```python
from build123d import *

# Parameters (mm, degrees)
F1_DEPTH       = 75
F2_T           = -0.01
F5_DEPTH       = 10
F6_DEPTH       = 10
F7_DEPTH       = 10
F8_DEPTH       = 10
F9_DEPTH       = 10
F10_DEPTH      = 10
F11_DEPTH      = 10
F12_DEPTH      = 10
F13_DEPTH      = 5
F4_E8_BOTTOM_W = 32
F4_E8_BOTTOM_H = 28
F14_DEPTH      = 0.01
F15_DEPTH      = 68


with BuildPart() as f1:
    # F0 (on Top) → F1 (new body)
    with BuildSketch(Plane.XY):
        Polygon((0, -147), (0, 0), (-70, 0), (-70, -45), (-135, -45), (-135, -96), (-120, -96), (-120, -147), align=None)
    extrude(amount=F1_DEPTH)

    # F2
    f2_openings = [f1.faces().sort_by_distance(p)[0] for p in [
        (-58.321727, -80.461003, 75),
    ]]
    offset(amount=F2_T, openings=f2_openings, kind=Kind.INTERSECTION)

    # F5 (add): a face of the model
    f5_faces = [f1.faces().sort_by_distance(p)[0] for p in [
        (0, -73.5, 37.5),
    ]]
    extrude(f5_faces, amount=F5_DEPTH)

    # F6 (add): a face of the model
    f6_faces = [f1.faces().sort_by_distance(p)[0] for p in [
        (-30, 0, 37.5),
    ]]
    extrude(f6_faces, amount=F6_DEPTH)

    # F7 (add): a face of the model
    f7_faces = [f1.faces().sort_by_distance(p)[0] for p in [
        (-70, -17.5, 37.5),
    ]]
    extrude(f7_faces, amount=F7_DEPTH)

    # F8 (add): a face of the model
    f8_faces = [f1.faces().sort_by_distance(p)[0] for p in [
        (-107.5, -45, 37.5),
    ]]
    extrude(f8_faces, amount=F8_DEPTH)

    # F9 (add): a face of the model
    f9_faces = [f1.faces().sort_by_distance(p)[0] for p in [
        (-135, -65.5, 37.5),
    ]]
    extrude(f9_faces, amount=F9_DEPTH)

    # F10 (add): a face of the model
    f10_faces = [f1.faces().sort_by_distance(p)[0] for p in [
        (-132.5, -96, 37.5),
    ]]
    extrude(f10_faces, amount=F10_DEPTH)

    # F11 (add): a face of the model
    f11_faces = [f1.faces().sort_by_distance(p)[0] for p in [
        (-120, -126.5, 37.5),
    ]]
    extrude(f11_faces, amount=F11_DEPTH)

    # F12 (add): a face of the model
    f12_faces = [f1.faces().sort_by_distance(p)[0] for p in [
        (-60, -147, 37.5),
    ]]
    extrude(f12_faces, amount=F12_DEPTH)

    # F13 (add): a face of the model
    f13_faces = [f1.faces().sort_by_distance(p)[0] for p in [
        (-59.1569047083, -79.5398738455, 0),
    ]]
    extrude(f13_faces, amount=F13_DEPTH)

    # F4_E8_bottom (on explicit) → F14 (join, through all)
    with BuildSketch(Plane(origin=(-134, -45, 0), x_dir=(1, 0, 0), z_dir=(0, 0, -1))):
        with Locations((16, 14)):
            Rectangle(F4_E8_BOTTOM_W, F4_E8_BOTTOM_H)
    extrude(amount=-F14_DEPTH)

    # F4_E8_bottom (on explicit) → F15 (join)
    with BuildSketch(Plane(origin=(-134, -45, 0), x_dir=(1, 0, 0), z_dir=(0, 0, -1))):
        with Locations((16, 14)):
            Rectangle(F4_E8_BOTTOM_W, F4_E8_BOTTOM_H)
    extrude(amount=-F15_DEPTH)


solid = f1.part
```
The model under review builds one solid part; all positions refer to its coordinate system, in mm. A direction names the side the tool comes from. Coordinates: 2 decimals unless noted, no trailing zeros. Order: outer loops, then holes, each group sorted by start corner. A loop starts at its lowest first (then second) coordinate and runs counter-clockwise, first axis right, second up. Notation, with made-up numbers: (-21.5, 38) -> (17.5, 38) arc R19 cw to (17.5, 61) -> close; hole circle Ø5 at (-4, -27). An arc over 180 degrees is marked (long way). Answer in a Markdown table with one row per item. Add a question column.
Item 1: Mouldability with a two-part tool opening along Y and no side actions: class faces 4 (the flat face through (-88, -45.01, 37)), 5 (the flat face through (-137, -106, 36)), 6 (the flat face through (-79, -42, 75)) as +Y half, -Y half, draft (parallel to the pull), parting line (faces both ways), or undercut.
Item 2: We need section B-B on x = -55.5. Write out the cut boundary in (y, z).
Item 3: Machinability: for faces 1 (the flat face through (-130, -131, 36)), 2 (the flat face through (-69.99, -22, 37)), 3 (the flat face through (-112, -35, 36)), which of the approach directions +Z, -Z, +X, -X, +Y, -Y give a long, thin tool a straight path to every point of the face, cutting with its end or side? Answer none if there is none.
Item 4: We need section A-A on y = -2.5. Write out the cut boundary in (x, z), plus the area to 3 significant figures.
Item 5: We need section C-C on z = 63. Write out the cut boundary in (x, y).
Item 6: To check wall thickness, follow probe 1 along Y at (x, z) = (-21, 30.5); probe 2 along X at (y, z) = (-60, 36.5); probe 3 along X at (y, z) = (-83, 49.5). State the ranges of each line that lie inside material, in increasing order.
Item 7: We need section D-D on x = -132. Write out the cut boundary in (y, z), plus the area to 3 significant figures.
Item 8: Clearance check with flat-ended pins moving along their axes: pin 1 (13.5 mm diameter, centred on y = -20.5, z = 40, fed in from -X); pin 2 (6 mm diameter, centred on x = -98, y = -64, fed in from +Z); pin 3 (4.5 mm diameter, centred on x = -124, z = 28.5, fed in from +Y). State where each tip first meets the part, or that it passes through.
Final values:
| question | item | result |
|---|---|---|
| 1 | face 4 | undercut |
| 1 | face 5 | -Y half |
| 1 | face 6 | draft |
| 2 | outline | (-157, -5) -> (10, -5) -> (10, 75) -> (-0.01, 75) -> (-0.01, 0.01) -> (-146.99, 0.01) -> (-146.99, 75) -> (-157, 75) -> close |
| 3 | face 1 | +Z, -Z, -X, -Y |
| 3 | face 2 | +Z |
| 3 | face 3 | +Z, -Z, -X, +Y |
| 4 | outline | (-80, -5) -> (10, -5) -> (10, 75) -> (-0.01, 75) -> (-0.01, 0.01) -> (-69.99, 0.01) -> (-69.99, 75) -> (-80, 75) -> close |
| 4 | area | 1,950 mm2 |
| 5 | outline | (-145, -106) -> (-130, -106) -> (-130, -157) -> (10, -157) -> (10, 10) -> (-80, 10) -> (-80, -35) -> (-145, -35) -> close; hole (-134.99, -95.99) -> (-119.99, -95.99) -> (-119.99, -146.99) -> (-0.01, -146.99) -> (-0.01, -0.01) -> (-69.99, -0.01) -> (-69.99, -45.01) -> (-102, -45.01) -> (-102, -73) -> (-134, -73) -> (-134, -45.01) -> (-134.99, -45.01) -> close |
| 6 | probe 1 | y = -157 to -146.99, -0.01 to 10 |
| 6 | probe 2 | x = -145 to -134.99, -134 to -102, -0.01 to 10 |
| 6 | probe 3 | x = -145 to -134.99, -0.01 to 10 |
| 7 | outline | (-106, -5) -> (-35, -5) -> (-35, 75) -> (-45.01, 75) -> (-45.01, 68) -> (-73, 68) -> (-73, 0.01) -> (-95.99, 0.01) -> (-95.99, 75) -> (-106, 75) -> close |
| 7 | area | 3,760 mm2 |
| 8 | pin 1 | stops at x = -80 |
| 8 | pin 2 | stops at z = 0.01 |
| 8 | pin 3 | stops at y = -35 |
